```python
from build123d import *

# Parameters (mm, degrees)
SKETCH1_W           = 90
SKETCH1_H           = 20
SKETCH1_R           = 2.65
SKETCH1_R_2         = 2.75
BOSS_EXTRUDE1_DEPTH = 20
CUT_EXTRUDE1_DEPTH  = 14
SKETCH3_R           = 4.5
CUT_EXTRUDE2_DEPTH  = 13


with BuildPart() as part:
    # Sketch1 → Boss-Extrude1 (new body)
    with BuildSketch(Plane(origin=(0, 0, 0), x_dir=(1, 0, 0), z_dir=(0, 1, 0))):
        Rectangle(SKETCH1_W, SKETCH1_H)
        with Locations(Location((-21, 0, 0), (0, 0, 270))):
            Circle(SKETCH1_R, mode=Mode.SUBTRACT)
        with Locations(Location((21, 0, 0), (0, 0, 270))):
            Circle(SKETCH1_R, mode=Mode.SUBTRACT)
        with Locations(Location((-37, 0, 0), (0, 0, 270))):
            Circle(SKETCH1_R_2, mode=Mode.SUBTRACT)
        with Locations(Location((37, 0, 0), (0, 0, 270))):
            Circle(SKETCH1_R_2, mode=Mode.SUBTRACT)
    extrude(amount=BOSS_EXTRUDE1_DEPTH)

    # Sketch2 → Cut-Extrude1 (cut)
    with BuildSketch(Plane.XZ):
        Polygon((-16.265727793, 0), (-18.632863896, 4.1), (-23.367136104, 4.1), (-25.734272207, 0), (-23.367136104, -4.1), (-18.632863896, -4.1), align=None)
        Polygon((25.734272207, 0), (23.367136104, 4.1), (18.632863896, 4.1), (16.265727793, 0), (18.632863896, -4.1), (23.367136104, -4.1), align=None)
    extrude(amount=-CUT_EXTRUDE1_DEPTH, mode=Mode.SUBTRACT)

    # Sketch3 → Cut-Extrude2 (cut)
    with BuildSketch(Plane(origin=(0, 20, 0), x_dir=(1, 0, 0), z_dir=(0, 1, 0))):
        with Locations(Location((-37, 0, 0), (0, 0, 270))):
            Circle(SKETCH3_R)
        with Locations(Location((37, 0, 0), (0, 0, 270))):
            Circle(SKETCH3_R)
    extrude(amount=-CUT_EXTRUDE2_DEPTH, mode=Mode.SUBTRACT)


solid = part.part
```
Check sheet for the modelled part. Datum: model origin and axes. Units: mm. A direction names the side the tool comes from. Round coordinates to 2 decimals unless told otherwise and drop trailing zeros. Write each loop counter-clockwise with the first axis right and the second up, starting at its lowest first coordinate (ties: lowest second). Pieces come first, ordered by that corner, then holes. Notation, with made-up numbers: M -31.75,81 L 21.25,81 A19 cw 21.25,92 Z; hole C -32,23.25 d7. An arc over 180 degrees is marked long. Write item = value, one per line. Start each with the question number.
1. Section check C-C, the plane y = 17. Record the cut outline in (x, z).
2. Section check A-A, the plane y = 6. Record the cut outline in (x, z).
3. Gauge pin test, flat ends, axial feed: pin 1 (8 mm diameter, centred on x = -37, z = 0, fed in from +Y); pin 2 (6 mm diameter, centred on x = 21, z = 0, fed in from -Y). Record the tip position at first contact, or that the pin passes through.
4. Release check for a two-part mould opening along Z. For faces 4 (the flat face through (17.466, 6.902, 2.079)), 5 (the flat face through (-21, 7, 4.1)), 6 (the flat face through (-1, 10, -10)), 7 (the flat face through (-1, 20, 0)) record: pulls with the +Z half, pulls with the -Z half, needs draft (parallel to the pull), parting line crosses it, or undercut.
5. Section check B-B, the plane x = -21. Record the cut outline in (y, z), then the cut area to 3 significant figures.
6. Scan lines: line 1 (X direction, y = 15.6, z = 0); line 2 (X direction, y = 4.75, z = -2.25); line 3 (Z direction, x = 37, y = 3). Record each from-to range of solid material in increasing order. Write a range as [from, to].
7. Tool access check on faces 1 (the flat face through (21, 7, -4.1)), 2 (the cylindrical face through (32.61, 13.59, -0.98)), 3 (the cylindrical face through (-18.37, 16.96, -0.34)). Record the directions out of +Z, -Z, +X, -X, +Y, -Y that give a thin tool (end or side, any length) a straight path to the whole face; none if there is none.
8. Section check D-D, the plane x = 24.5. Record the cut outline in (y, z), then the cut area to 3 significant figures.
Results found:
q1.outline = M -45,-10 L 45,-10 L 45,10 L -45,10 Z; hole C -37,0 d9; hole C -21,0 d5.3; hole C 21,0 d5.3; hole C 37,0 d9
q2.outline = M -45,-10 L 45,-10 L 45,10 L -45,10 Z; hole C -37,0 d5.5; hole M -25.73,0 L -23.37,-4.1 L -18.63,-4.1 L -16.27,0 L -18.63,4.1 L -23.37,4.1 Z; hole M 16.27,0 L 18.63,-4.1 L 23.37,-4.1 L 25.73,0 L 23.37,4.1 L 18.63,4.1 Z; hole C 37,0 d5.5
q3.pin_1 = 7
q3.pin_2 = 14
q4.face_4 = undercut
q4.face_5 = undercut
q4.face_6 = pulls with the -Z half
q4.face_7 = needs draft
q5.outline = M 0,-10 L 20,-10 L 20,-2.65 L 14,-2.65 L 14,-4.1 L 0,-4.1 Z; M 0,4.1 L 14,4.1 L 14,2.65 L 20,2.65 L 20,10 L 0,10 Z
q5.area = 253 mm^2
q6.line_1 = [-45, -41.5], [-32.5, -23.65], [-18.35, 18.35], [23.65, 32.5], [41.5, 45]
q6.line_2 = [-45, -38.58], [-35.42, -24.44], [-17.56, 17.56], [24.44, 35.42], [38.58, 45]
q6.line_3 = [-10, -2.75], [2.75, 10]
q7.face_1 = -Y
q7.face_2 = +Y
q7.face_3 = +Y, -Y
q8.outline = M 0,-10 L 20,-10 L 20,10 L 0,10 L 0,2.14 L 14,2.14 L 14,-2.14 L 0,-2.14 Z
q8.area = 340 mm^2
